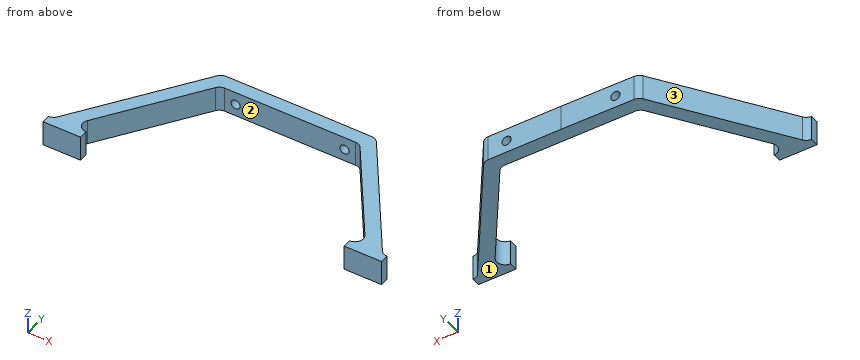
from build123d import *

# Parameters (mm, degrees)
F1_DEPTH = 9
F2_R     = 1.65
F3_DEPTH = 25


with BuildPart() as f1:
    # F0 (on Top) → F1 (new body)
    with BuildSketch(Plane.XY):
        with BuildLine():
            Line((-49.702811, -40.279271), (-25.895755, -6.279271))
            ThreePointArc((-25.895755, -6.279271), (-24.823545, -5.338968), (-23.438299, -5))
            Line((-23.438299, -5), (0, -5))
            Line((0, -5), (23.438299, -5))
            ThreePointArc((23.438299, -5), (24.823545, -5.338968), (25.895755, -6.279271))
            Line((25.895755, -6.279271), (49.702811, -40.279271))
            ThreePointArc((49.702811, -40.279271), (49.906388, -43.385246), (47.245355, -45))
            Line((47.245355, -45), (47.245355, -48))
            Line((47.245355, -48), (60.673876, -48))
            Line((60.673876, -48), (60.673876, -45))
            ThreePointArc((60.673876, -45), (59.28863, -44.661032), (58.216419, -43.720729))
            Line((58.216419, -43.720729), (28.588166, -1.407198))
            ThreePointArc((28.588166, -1.407198), (27.522463, -0.470292), (26.145392, -0.127963))
            Line((26.145392, -0.127963), (0, 0))
            Line((0, 0), (-26.145392, -0.127963))
            ThreePointArc((-26.145392, -0.127963), (-27.522463, -0.470292), (-28.588166, -1.407198))
            Line((-28.588166, -1.407198), (-58.216419, -43.720729))
            ThreePointArc((-58.216419, -43.720729), (-59.28863, -44.661032), (-60.673876, -45))
            Line((-60.673876, -45), (-60.673876, -48))
            Line((-60.673876, -48), (-47.245355, -48))
            Line((-47.245355, -48), (-47.245355, -45))
            ThreePointArc((-47.245355, -45), (-49.906388, -43.385246), (-49.702811, -40.279271))
        make_face()
    extrude(amount=F1_DEPTH)

    # F2 (on face) → F3 (cut)
    with BuildSketch(Plane(origin=(0, 0, 0), x_dir=(-0.999988, 0.004894, 0), z_dir=(0.004894, 0.999988, 0))):
        with Locations((-19.5, 4.371774)):
            Circle(F2_R)
        with Locations((19.5, 4.371774)):
            Circle(F2_R)
    extrude(amount=-F3_DEPTH, mode=Mode.SUBTRACT)


solid = f1.part
Model file for the job. Use its own axes, mm. Face numbers are marked on the shaded views. Give positions to 0.01 mm unless a question says otherwise; leave off trailing zeros. Order: outer loops, then holes, each group sorted by start corner. A loop starts at its lowest first (then second) coordinate and runs counter-clockwise, first axis right, second up. Notation, with made-up numbers: (74.5, 74) - (91.5, 74) arc R33 cw to (91.5, 112) - close; hole circle Ø5 at (75.5, 49). An arc over 180 degrees is marked (long way). Return JSON: item names as keys, results as strings.
1) Pull direction X, two halves, no side cores. Call the marked faces 1, 2 and 3: pulls with the +X half, pulls with the -X half, needs draft (parallel to the pull), parting line crosses it, or undercut.
Geometry says:
{"face 1": "needs draft", "face 2": "undercut", "face 3": "pulls with the -X half"}
2) Cut at C-C, the plane x = 9.5. Give the cut face in (y, z), plus the area to 3 significant figures.
Geometry says:
{"outline": "(-5, 0) - (-0.05, 0) - (-0.05, 9) - (-5, 9) - close", "area": "44.6 mm²"}
3) Probe line 1 (X direction, y = -46, z = 5.25); line 2 (Y direction, x = 22, z = 1.25); line 3 (Y direction, x = 1, z = 2.5). List the from-to ranges inside material, lowest first. Write a range as from..to.
Geometry says:
{"line 1": "-60.67..-47.25, 47.25..60.67", "line 2": "-5..-0.11", "line 3": "-5..0"}
4) Flat gauge pins, fed straight in: P1, Ø1, axis at x = -13.5, z = 4.5, coming from the +Y side; P2, Ø2.5, axis at x = -3.5, z = 6.5, coming from the -Y side; P3, Ø3, axis at y = -26, z = 7, coming from the +X side. Where does each tip first touch, or does it go through?
Geometry says:
{"P1": "y = -0.06", "P2": "y = -5", "P3": "x = 46.86"}
5) Cut at A-A, the plane z = 1.5. Give the cut face in (x, y).
Geometry says:
{"outline": "(-60.67, -48) - (-47.25, -48) - (-47.25, -45) arc R3 cw to (-49.7, -40.28) - (-25.9, -6.28) arc R3 cw to (-23.44, -5) - (23.44, -5) arc R3 cw to (25.9, -6.28) - (49.7, -40.28) arc R3 cw to (47.25, -45) - (47.25, -48) - (60.67, -48) - (60.67, -45) arc R3 cw to (58.22, -43.72) - (28.59, -1.41) arc R3 ccw to (26.15, -0.13) - (0, 0) - (-26.15, -0.13) arc R3 ccw to (-28.59, -1.41) - (-58.22, -43.72) arc R3 cw to (-60.67, -45) - close"}
6) Cut at B-B, the plane y = -33.5. Give the cut face in (x, z), plus the area to 3 significant figures.
Geometry says:
{"outline": "(-51.06, 0) - (-44.96, 0) - (-44.96, 9) - (-51.06, 9) - close; (44.96, 0) - (51.06, 0) - (51.06, 9) - (44.96, 9) - close", "area": "110 mm²"}
